Geometry check sheet. Reference: drawing and pictorial views, mm from the part's lowest x, y, z. Coordinates: 2 decimals unless noted, no trailing zeros. Loops run counter-clockwise (first coordinate to the right, second up) from the corner with the lowest first, then second, coordinate; pieces in that order, holes last. Notation, with made-up numbers: (44.25, -17.5) -> (75.25, -17.5) arc R14 cw to (75.25, 4.5) -> close; hole circle Ø5 at (-7, 7). An arc over 180 degrees is marked (long way). Answer as a JSON object with one key per item and string values. Group by question number.
Q1. Gauge pin test, flat end, axial feed: pin 1 Ø13 at (x, y) = (18, 81.56) entering from -Z. Record the tip position at first contact, or that the pin passes through.
Q2. Cross-section at C-C on x = 85. Record the boundary of the cut face in (y, z).
Q3. Cross-section at A-A on x = 18. Record the boundary of the cut face in (y, z), and give its area (3 significant figures).
Q4. Cross-section at B-B on y = 7. Record the boundary of the cut face in (x, z), and give its area (3 significant figures).
Q5. Scan lines: L1, parallel to X at y = 82, z = 4.75; L2, parallel to Y at x = 18, z = 3.25; L3, parallel to Y at x = 85, z = 4.5. Record each from-to range of solid material in increasing order.
Q6. Cross-section at D-D on y = 81.56. Record the boundary of the cut face in (x, z).
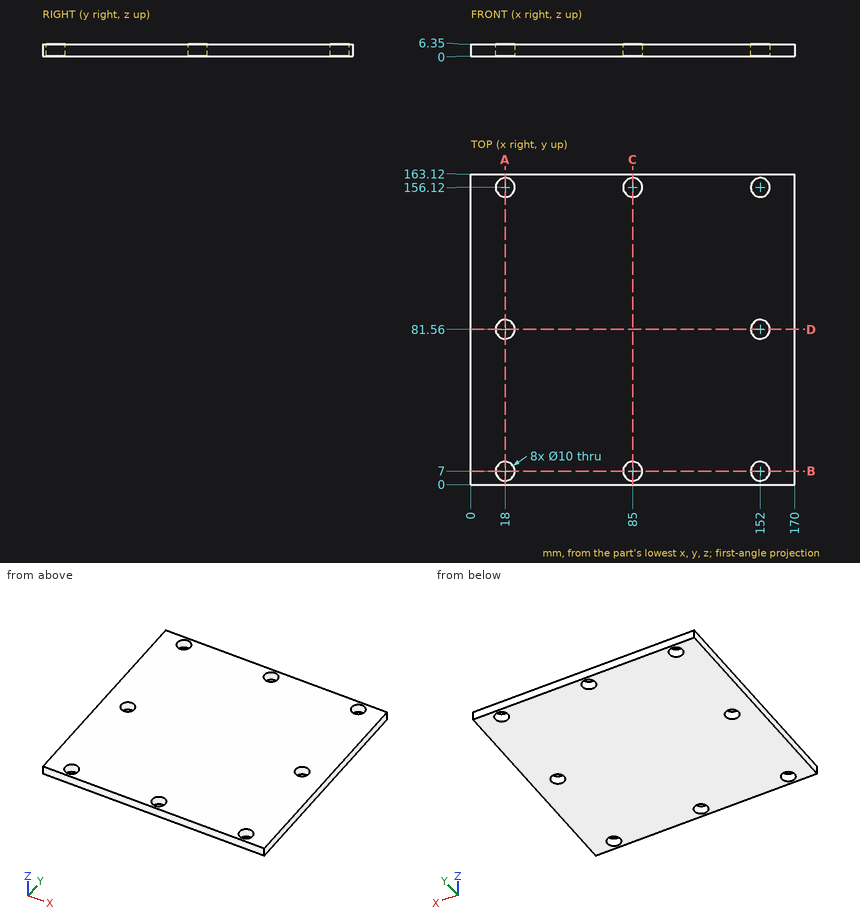
Computed values:
{
 "1": {"pin 1": "stops at z = 0"},
 "2": {"outline": "(0, 0) -> (2, 0) -> (2, 6.35) -> (0, 6.35) -> close; (12, 0) -> (151.12, 0) -> (151.12, 6.35) -> (12, 6.35) -> close; (161.12, 0) -> (163.12, 0) -> (163.12, 6.35) -> (161.12, 6.35) -> close"},
 "3": {"outline": "(0, 0) -> (2, 0) -> (2, 6.35) -> (0, 6.35) -> close; (12, 0) -> (76.56, 0) -> (76.56, 6.35) -> (12, 6.35) -> close; (86.56, 0) -> (151.12, 0) -> (151.12, 6.35) -> (86.56, 6.35) -> close; (161.12, 0) -> (163.12, 0) -> (163.12, 6.35) -> (161.12, 6.35) -> close", "area": "845 mm²"},
 "4": {"outline": "(0, 0) -> (13, 0) -> (13, 6.35) -> (0, 6.35) -> close; (23, 0) -> (80, 0) -> (80, 6.35) -> (23, 6.35) -> close; (90, 0) -> (147, 0) -> (147, 6.35) -> (90, 6.35) -> close; (157, 0) -> (170, 0) -> (170, 6.35) -> (157, 6.35) -> close", "area": "889 mm²"},
 "5": {"L1": "x = 0 to 13.02, 22.98 to 147.02, 156.98 to 170", "L2": "y = 0 to 2, 12 to 76.56, 86.56 to 151.12, 161.12 to 163.12", "L3": "y = 0 to 2, 12 to 151.12, 161.12 to 163.12"},
 "6": {"outline": "(0, 0) -> (13, 0) -> (13, 6.35) -> (0, 6.35) -> close; (23, 0) -> (147, 0) -> (147, 6.35) -> (23, 6.35) -> close; (157, 0) -> (170, 0) -> (170, 6.35) -> (157, 6.35) -> close"}
}
